Part model, mm, in its own coordinate system. Coordinates: 2 decimals unless noted, no trailing zeros. Order: outer loops, then holes, each group sorted by start corner. A loop starts at its lowest first (then second) coordinate and runs counter-clockwise, first axis right, second up.
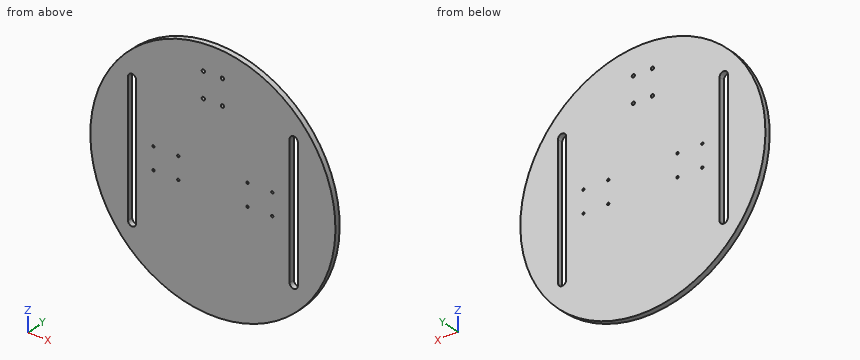
```python
from build123d import *

# Parameters (mm, degrees)
SKETCH1_R           = 225
SKETCH1_R_2         = 3
BOSS_EXTRUDE1_DEPTH = 10
SKETCH3_R           = 2.1
CUT_EXTRUDE2_DEPTH  = 10


with BuildPart() as part:
    # Sketch1 → Boss-Extrude1 (new body)
    with BuildSketch(Plane(origin=(0, 0, 0), x_dir=(1, 0, 0), z_dir=(0, 1, 0))):
        with Locations(Location((0, 0, 0), (0, 0, 270))):
            Circle(SKETCH1_R)
        with Locations(Location((-17.5, -132.051038191, 0), (0, 0, 270))):
            Circle(SKETCH1_R_2, mode=Mode.SUBTRACT)
        with Locations(Location((17.5, -132.051038191, 0), (0, 0, 270))):
            Circle(SKETCH1_R_2, mode=Mode.SUBTRACT)
        with Locations(Location((17.5, -178.051038191, 0), (0, 0, 270))):
            Circle(SKETCH1_R_2, mode=Mode.SUBTRACT)
        with Locations(Location((-17.5, -178.051038191, 0), (0, 0, 270))):
            Circle(SKETCH1_R_2, mode=Mode.SUBTRACT)
        with BuildLine():
            Line((-155.90685468, -120), (-155.90685468, 120))
            ThreePointArc((-155.90685468, 120), (-148.40685468, 127.5), (-140.90685468, 120))
            Line((-140.90685468, 120), (-140.90685468, -120))
            ThreePointArc((-140.90685468, -120), (-148.40685468, -127.5), (-155.90685468, -120))
        make_face(mode=Mode.SUBTRACT)
        with BuildLine():
            Line((155.90685468, -120), (155.90685468, 120))
            ThreePointArc((155.90685468, 120), (148.40685468, 127.5), (140.90685468, 120))
            Line((140.90685468, 120), (140.90685468, -120))
            ThreePointArc((140.90685468, -120), (148.40685468, -127.5), (155.90685468, -120))
        make_face(mode=Mode.SUBTRACT)
    extrude(amount=BOSS_EXTRUDE1_DEPTH)

    # Sketch3 → Cut-Extrude2 (cut)
    with BuildSketch(Plane(origin=(0, 10, 0), x_dir=(1, 0, 0), z_dir=(0, 1, 0))):
        with Locations(Location((63.533017038, -20, 0), (0, 0, 270))):
            Circle(SKETCH3_R)
        with Locations(Location((63.533017038, 20, 0), (0, 0, 270))):
            Circle(SKETCH3_R)
        with Locations(Location((-63.533017038, -20, 0), (0, 0, 90))):
            Circle(SKETCH3_R)
        with Locations(Location((-109.034473384, -20, 0), (0, 0, 270))):
            Circle(SKETCH3_R)
        with Locations(Location((-63.533017038, 20, 0), (0, 0, 270))):
            Circle(SKETCH3_R)
        with Locations(Location((-109.034473384, 20, 0), (0, 0, 90))):
            Circle(SKETCH3_R)
        with Locations(Location((109.034473384, -20, 0), (0, 0, 90))):
            Circle(SKETCH3_R)
        with Locations(Location((109.034473384, 20, 0), (0, 0, 270))):
            Circle(SKETCH3_R)
    extrude(amount=-CUT_EXTRUDE2_DEPTH, mode=Mode.SUBTRACT)


solid = part.part
```
(1) Drop flat-ended pins along their axis: pin 1 (2.5 mm diameter, centred on x = 63.53, z = -20, fed in from -Y) (1 decimal); pin 2 (3 mm diameter, centred on x = -14.5, y = 4, fed in from -Z). Give the stop position or say it passes through.
(2) Slice it at C-C, the plane x = -98.5. Give the cut face in (y, z).
(3) Slice it at A-A, the plane y = 2.25. State how many separate pieces and enclosed holes the cut face has, then the cut area to 3 significant figures.
(4) Slice it at B-B, the plane z = 113. Give the cut face in (x, y).
(5) Slice it at D-D, the plane x = 100.5. Give the cut face in (y, z), then the cut area to 3 significant figures.
(6) Probe line 1 (X direction, y = 3, z = 58.5); line 2 (X direction, y = 7.5, z = -15); line 3 (Z direction, x = -64.5, y = 7.75). List the from-to ranges inside material, lowest first.
Here are the results:
1. pin 1: passes through
1. pin 2: stops at z = -224.62
2. outline: (0, -202.29) - (10, -202.29) - (10, 202.29) - (0, 202.29) - close
3. separate pieces: 1
3. enclosed holes: 14
3. area: 151,000 mm2
4. outline: (-194.57, 0) - (-155.91, 0) - (-155.91, 10) - (-194.57, 10) - close; (-140.91, 0) - (140.91, 0) - (140.91, 10) - (-140.91, 10) - close; (155.91, 0) - (194.57, 0) - (194.57, 10) - (155.91, 10) - close
5. outline: (0, -201.31) - (10, -201.31) - (10, 201.31) - (0, 201.31) - close
5. area: 4,030 mm2
6. line 1: x = -217.26 to -155.91, -140.91 to 140.91, 155.91 to 217.26
6. line 2: x = -224.5 to -155.91, -140.91 to 140.91, 155.91 to 224.5
6. line 3: z = -215.56 to -21.86, -18.14 to 18.14, 21.86 to 215.56
